Autodesk Inventor part; units mm, degrees
ref_plane "YZ Plane (RIGHT)" through (0, 0, 0) normal (1, 0, 0) x (0, 1, 0)
ref_plane "XZ Plane (TOP)" through (0, 0, 0) normal (0, 1, 0) x (-1, 0, 0)
ref_plane "XY Plane (FRONT)" through (0, 0, 0) normal (0, 0, 1) x (1, 0, 0)
sketch "Sketch2" plane through (0, 0, 0) normal (0, 0, 1) x (1, 0, 0)
  line L0 (-4.445, 0) -> (4.445, 0) construction
  line L1 (0, 9.8146) -> (0, -1.6358) construction
  line L2 (-3.175, 0) -> (3.175, 0)
  line L3 (2.159, 3.175) -> (-3.175, 3.175)
  line L4 (-3.175, 3.175) -> (-3.175, 0)
  line L5 (3.175, 0) -> (3.175, 8.1788)
  line L6 (3.175, 8.1788) -> (2.159, 8.1788)
  line L7 (2.159, 8.1788) -> (1.4478, 6.5607)
  line L8 (1.4478, 6.5607) -> (2.159, 4.9425)
  line L9 (2.159, 4.9425) -> (2.159, 3.175)
  point P0 (0, 0)
  dimension "d0" = 6.35
  dimension "d1" = 3.175
  dimension "d2" = 8.1788
  dimension "d3" = 1.4478
  dimension "d4" = 1.016
extrude "Extrusion1" add sketch "Sketch2" along normal mid plane 2.54
sketch "Sketch3" plane through (-3.175, 0, 1.27) normal (0, -1, 0) x (1, 0, 0)
  line L0 (-1.27, -1.27) -> (7.62, -1.27) construction
  line L1 (3.175, 0.508) -> (3.175, -3.048) construction
  line L2 (2.794, -0.889) -> (3.556, -0.889)
  line L3 (3.556, -0.889) -> (3.556, -1.651)
  line L4 (3.556, -1.651) -> (2.794, -1.651)
  line L5 (2.794, -1.651) -> (2.794, -0.889)
  circle A0 centre (3.175, -1.27) radius 0.4445
  dimension "d7" = 0.762
  dimension "d15" = 0.889
extrude "Extrusion2" add sketch "Sketch3" along normal blind 2.794 contours A0 L2 | L2 A0 L3 L4 L5 | L5 A0 | A0 L3 | L4 A0
extrude "Extrusion3" add sketch "Sketch3" against normal blind 10.668 contours L2 A0 L5 | L2 A0 L3 L4 L5 | L2 L3 A0 | A0 L4 L5 | L3 L4 A0
pattern_linear "Rectangular Pattern1" count 2 spacing 2.54 along (0, 0, 1) of "Extrusion1", "Extrusion2", "Extrusion3"
properties part number "Molex KK 2 Pin"
Verification items for the finished model (mm, model axes). A direction names the side the tool comes from. Round coordinates to 2 decimals unless told otherwise and drop trailing zeros. Loops run counter-clockwise (first coordinate to the right, second up) from the corner with the lowest first, then second, coordinate; pieces in that order, holes last. Notation, with made-up numbers: (-36, 81.5) - (-9, 81.5) arc R29 cw to (-9, 110.5) - close; hole circle Ø2 at (-9, 74). An arc over 180 degrees is marked (long way). Use a Markdown table: item, result. Add a question column.
1. Access from +Z, -Z, +X, -X, +Y, -Y to the whole of each face (thin tool, end or side, straight path). Record for faces 5 (the face through (3, 8.179, 1)), 6 (the face through (1.81, 7.38, 1.23)), 7 (the face through (1, 2, -1.27)), 8 (the face through (-0.06, -1.38, 2.1)), 9 (the face through (3.175, 4, 1)).
2. Section check C-C, the plane z = 1.8. Record the boundary of the cut face in (x, y) (1 decimal).
3. Section check B-B, the plane x = 0. Record the boundary of the cut face in (y, z) (1 decimal), plus the area to 3 significant figures.
4. Gauge pin test, flat ends, axial feed: pin 1 (0.6 mm diameter, centred on y = 8.5, z = 2.5, fed in from -X); pin 2 (0.8 mm diameter, centred on x = 0, y = 7, fed in from -Z); pin 3 (0.6 mm diameter, centred on x = 0, y = 8.5, fed in from +Z); pin 4 (1 mm diameter, centred on x = -1, y = 4.5, fed in from -Z). Record the tip position at first contact, or that the pin passes through.
5. Thickness scan on probe 1 along Z at (x, y) = (-0.25, 3.5); probe 2 along X at (y, z) = (3.75, -0.35) (3 decimals); probe 3 along Y at (x, z) = (0.5, 0.1) (3 decimals). Record the ranges inside material, lowest first. Write a range as [from, to].
6. Section check D-D, the plane y = 4.5. Record the boundary of the cut face in (x, z) (3 decimals), plus the area to 3 significant figures.
7. Release check for a two-part mould opening along Y. For faces 1 (the face through (-0.096, -1.377, 0.434)), 2 (the face through (0, -2.794, 0)), 3 (the face through (2.159, 4, 1)), 4 (the face through (1.8, 5.76, 1.23)) record: released by +Y, released by -Y, zero draft, split by the parting line, or undercut.
8. Section check A-A, the plane y = 8.5. Record the boundary of the cut face in (x, z), plus the area to 3 significant figures.
Checks:
| question | item | result |
|---|---|---|
| 1 | face 5 | +Z, -Z, +X, +Y |
| 1 | face 6 | +Z, -Z, +Y |
| 1 | face 7 | -Z, +X, -X, +Y, -Y |
| 1 | face 8 | -Y |
| 1 | face 9 | +Z, -Z, +X, +Y, -Y |
| 2 | outline | (-3.2, 0) - (3.2, 0) - (3.2, 8.2) - (2.2, 8.2) - (1.4, 6.6) - (2.2, 4.9) - (2.2, 3.2) - (-3.2, 3.2) - close |
| 3 | outline | (-2.8, -0.4) - (0, -0.4) - (0, -1.3) - (3.2, -1.3) - (3.2, -0.4) - (10.7, -0.4) - (10.7, 0.4) - (3.2, 0.4) - (3.2, 2.2) - (10.7, 2.2) - (10.7, 2.9) - (3.2, 2.9) - (3.2, 3.8) - (0, 3.8) - (0, 3) - (-2.8, 3) - (-2.8, 2.1) - (0, 2.1) - (0, 0.4) - (-2.8, 0.4) - close |
| 3 | area | 32.5 mm^2 |
| 4 | pin 1 | stops at x = -0.38 |
| 4 | pin 2 | stops at z = -0.38 |
| 4 | pin 3 | stops at z = 2.92 |
| 4 | pin 4 | passes through |
| 5 | probe 1 | z = [-0.38, 0.38], [2.16, 2.92] |
| 5 | probe 2 | x = [-0.381, 0.381], [2.159, 3.175] |
| 5 | probe 3 | y = [0, 3.175] |
| 6 | outline | (-0.381, -0.381) - (0.381, -0.381) - (0.381, 0.381) - (-0.381, 0.381) - close; (-0.381, 2.159) - (0.381, 2.159) - (0.381, 2.921) - (-0.381, 2.921) - close; (2.159, -1.27) - (3.175, -1.27) - (3.175, 3.81) - (2.159, 3.81) - close |
| 6 | area | 6.32 mm^2 |
| 7 | face 1 | zero draft |
| 7 | face 2 | released by -Y |
| 7 | face 3 | undercut |
| 7 | face 4 | undercut |
| 8 | outline | (-0.38, -0.38) - (0.38, -0.38) - (0.38, 0.38) - (-0.38, 0.38) - close; (-0.38, 2.16) - (0.38, 2.16) - (0.38, 2.92) - (-0.38, 2.92) - close |
| 8 | area | 1.16 mm^2 |
